Here's how the part is built. I have some questions about the finished solid (model axes, mm). A direction names the side the tool comes from. Coordinates: 2 decimals unless noted, no trailing zeros. Write each loop counter-clockwise with the first axis right and the second up, starting at its lowest first coordinate (ties: lowest second). Pieces come first, ordered by that corner, then holes. Notation, with made-up numbers: M 13,78 L 47,78 A23 ccw 47,105 Z; hole C 30.25,7 d10. An arc over 180 degrees is marked long. Use one line per item in the form item = value. Start each with the question number.
1. I want a section at C-C, the plane z = 8. List the corners of the cut face in (x, y) for me, plus the area to 3 significant figures.
2. I want a section at B-B, the plane y = 18.5. List the corners of the cut face in (x, z) for me, plus the area to 3 significant figures.
3. Thinking about a two-plate mould opening in Y: for faces 1 (the face through (4.278, 2.752, 10.713)), 2 (the face through (-4.222, 11.264, 0.385)), 3 (the face through (-4, 9, 10)), which applies, released by +Y, released by -Y, zero draft, split by the parting line, or undercut?
4. I'm going to push flat-ended pins straight in: pin 1 Ø2 at (y, z) = (5.5, -6) entering from +X; pin 2 Ø6.5 at (y, z) = (13, 3.5) entering from -X; pin 3 Ø1.5 at (x, z) = (9, 8.5) entering from +Y; pin 4 Ø5 at (y, z) = (15.5, 13) entering from -X. Where does each tip first touch, or does it pass through?
5. On a 3-axis mill with a long thin cutter (end or side, diameter ignored), from which of +Z, -Z, +X, -X, +Y, -Y can I reach the whole of each face in a straight line? I mean faces 4 (the face through (2.25, 10, 0)), 5 (the face through (-6.25, 10, 0)), 6 (the face through (-4, 9, -10)), 7 (the face through (6.25, 10, 0)). Say none if no direction works.
6. I want a section at D-D, the plane x = -7.5. List the corners of the cut face in (y, z) for me.
7. I want a section at A-A, the plane z = 0. List the corners of the cut face in (x, y) for me, plus the area to 3 significant figures.
8. Please list where these lines run through material, in increasing order: line 1 along Y through (x, z) = (5.3, 0); line 2 along X through (y, z) = (14, 8.5); line 3 along Y through (x, z) = (12.5, -15.5). Write a range as [from, to].
from build123d import *

# Parameters (mm, degrees)
ESQUISSE1_W             = 30
ESQUISSE1_H             = 40
BOSS_EXTRU_1_DEPTH      = 2
ESQUISSE2_W             = 4
ESQUISSE2_H             = 20
BOSS_EXTRU_2_DEPTH      = 11
BOSS_EXTRU_3_START      = -4
BOSS_EXTRU_3_DEPTH      = 4
BOSS_EXTRU_4_START      = -4
BOSS_EXTRU_4_DEPTH      = 4
ESQUISSE5_R             = 1.778
ENL_V_MAT_EXTRU_1_DEPTH = 12.5
CONG_1_R                = 2.5


with BuildPart() as part:
    # Esquisse1 → Boss.-Extru.1 (new body)
    with BuildSketch(Plane(origin=(0, 0, 0), x_dir=(1, 0, 0), z_dir=(0, 1, 0))):
        Rectangle(ESQUISSE1_W, ESQUISSE1_H)
    extrude(amount=BOSS_EXTRU_1_DEPTH)

    # Esquisse2 → Boss.-Extru.2 (add)
    with BuildSketch(Plane(origin=(0, 2, 0), x_dir=(1, 0, 0), z_dir=(0, 1, 0))):
        with Locations((4.25, 0)):
            Rectangle(ESQUISSE2_W, ESQUISSE2_H)
        with Locations((-4.25, 0)):
            Rectangle(ESQUISSE2_W, ESQUISSE2_H)
    extrude(amount=BOSS_EXTRU_2_DEPTH)

    # Esquisse3 → Boss.-Extru.3 (add)
    with BuildSketch(Plane.ZY.offset(6.25).offset(BOSS_EXTRU_3_START)):
        with BuildLine():
            Line((-10, 13), (10, 13))
            ThreePointArc((10, 13), (0, 23), (-10, 13))
        make_face()
    extrude(amount=BOSS_EXTRU_3_DEPTH)

    # Esquisse4 → Boss.-Extru.4 (add)
    with BuildSketch(Plane(origin=(6.25, 0, 0), x_dir=(0, 0, -1), z_dir=(1, 0, 0)).offset(BOSS_EXTRU_4_START)):
        with BuildLine():
            Line((10, 13), (-10, 13))
            ThreePointArc((-10, 13), (0, 23), (10, 13))
        make_face()
    extrude(amount=BOSS_EXTRU_4_DEPTH)

    # Esquisse5 → Enlèv. mat.-Extru.1 (cut)
    with BuildSketch(Plane(origin=(6.25, 0, 0), x_dir=(0, 0, -1), z_dir=(1, 0, 0))):
        with Locations((0, 13)):
            Circle(ESQUISSE5_R)
    extrude(amount=-ENL_V_MAT_EXTRU_1_DEPTH, mode=Mode.SUBTRACT)

    # Congé1
    cong_1_edges = [part.edges().sort_by_distance(p)[0] for p in [
        (4.25, 2, 10),
        (4.25, 2, -10),
        (-4.25, 2, -10),
        (-4.25, 2, 10),
        (-15, 1, -20),
        (15, 1, -20),
        (15, 1, 20),
        (-15, 1, 20),
    ]]
    fillet(cong_1_edges, radius=CONG_1_R)


solid = part.part
Answer list:
q1.outline = M -15,0 L 15,0 L 15,2 L 6.25,2 L 6.25,19 L 2.25,19 L 2.25,2 L -2.25,2 L -2.25,19 L -6.25,19 L -6.25,2 L -15,2 Z
q1.area = 196 mm²
q2.outline = M -6.25,-8.35 L -2.25,-8.35 L -2.25,8.35 L -6.25,8.35 Z; M 2.25,-8.35 L 6.25,-8.35 L 6.25,8.35 L 2.25,8.35 Z
q2.area = 134 mm²
q3.face_1 = released by +Y
q3.face_2 = undercut
q3.face_3 = zero draft
q4.pin_1 = 6.25
q4.pin_2 = -6.25
q4.pin_3 = 2
q4.pin_4 = through
q5.face_4 = +Z, -Z, +Y
q5.face_5 = +Z, -Z, -X, +Y
q5.face_6 = -Z, +X, -X, +Y
q5.face_7 = +Z, -Z, +X, +Y
q6.outline = M 0,-20 L 2,-20 L 2,20 L 0,20 Z
q7.outline = M -15,0 L 15,0 L 15,2 L 6.25,2 L 6.25,11.22 L 2.25,11.22 L 2.25,2 L -2.25,2 L -2.25,11.22 L -6.25,11.22 L -6.25,2 L -15,2 Z; M -6.25,14.78 L -2.25,14.78 L -2.25,23 L -6.25,23 Z; M 2.25,14.78 L 6.25,14.78 L 6.25,23 L 2.25,23 Z
q7.area = 200 mm²
q8.line_1 = [0, 11.22], [14.78, 23]
q8.line_2 = [-6.25, -2.25], [2.25, 6.25]
q8.line_3 = [0, 2]
